The drawing under review shows one solid part. Ordinate dimensions are in mm from its lowest x, y, z. A direction names the side the tool comes from. Round coordinates to 2 decimals unless told otherwise and drop trailing zeros. Order: outer loops, then holes, each group sorted by start corner. A loop starts at its lowest first (then second) coordinate and runs counter-clockwise, first axis right, second up. Notation, with made-up numbers: M -32.5,67.5 L 26.5,67.5 A19 ccw 26.5,95.5 Z; hole C -8.5,-13.5 d7. An arc over 180 degrees is marked long. Answer as a JSON object with one key per item and string values. Group by question number.
1) The part is to be moulded in two halves that separate along X. For the marked faces 1, 2 and 3, say which applies: +X half, -X half, draft (parallel to the pull), parting line (faces both ways), or undercut.
2) For the marked faces 4 and 5, list the 3-axis set-ups (+Z, -Z, +X, -X, +Y, -Y) from which the entire face can be reached by the end or side of a thin tool; tool diameter is ignored.
3) Consider section A-A, the plane z = 4.5. Write out the cut boundary in (x, y) (1 decimal).
4) Insertion check: pin 1 Ø1 at (y, z) = (3.5, 0.5) entering from -X; pin 2 Ø1.5 at (y, z) = (3, 1) entering from +X (1 decimal). Each pin has a flat end and moves straight along its axis. Give the tip position at first contact, or say it passes through.
5) To check wall thickness, follow line 1 (Y direction, x = 5.5, z = 3.25) (1 decimal); line 2 (Z direction, x = 0.5, y = 6) (1 decimal). State the ranges of each line that lie inside material, in increasing order.
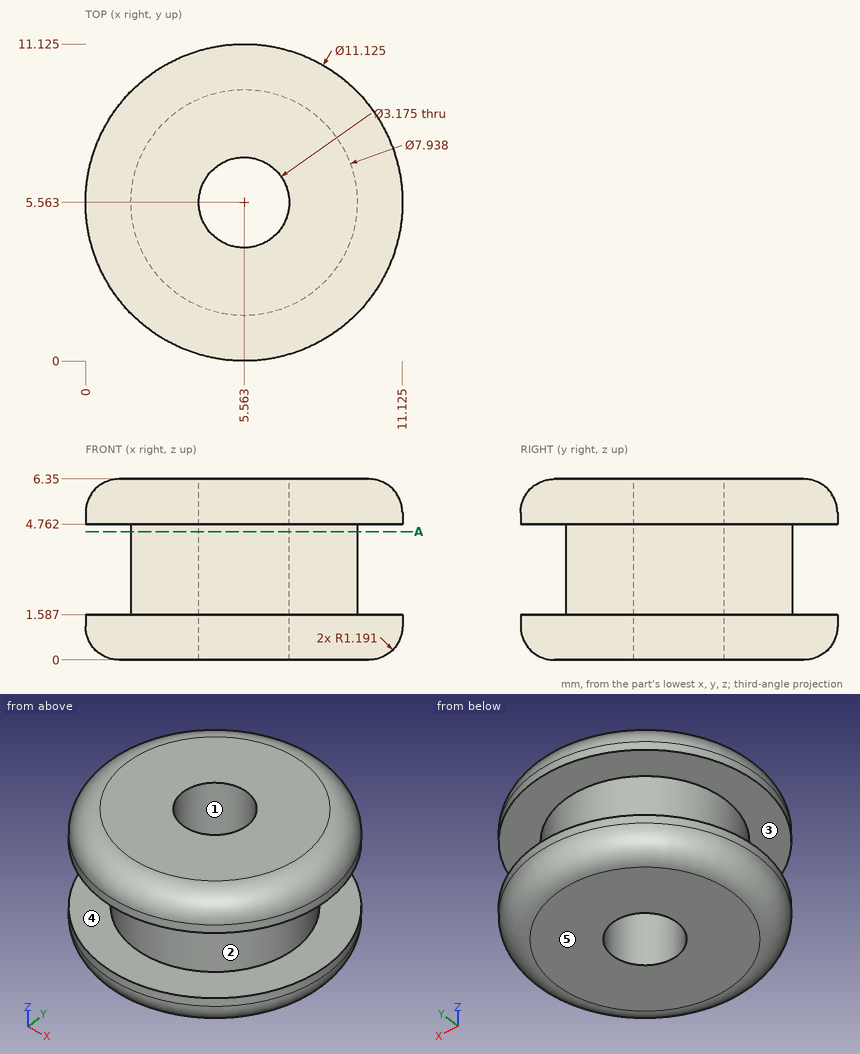
Results list:
{
 "1": {"face 1": "undercut", "face 2": "parting line", "face 3": "draft"},
 "2": {"face 4": "none", "face 5": "-Z, +X, -X, +Y, -Y"},
 "3": {"outline": "C 5.6,5.6 d7.9; hole C 5.6,5.6 d3.2"},
 "4": {"pin 1": "x = 0.32", "pin 2": "x = 10.8"},
 "5": {"line 1": "1.6 to 4, 7.1 to 9.5", "line 2": "0.2 to 1.6, 4.8 to 6.1"}
}
